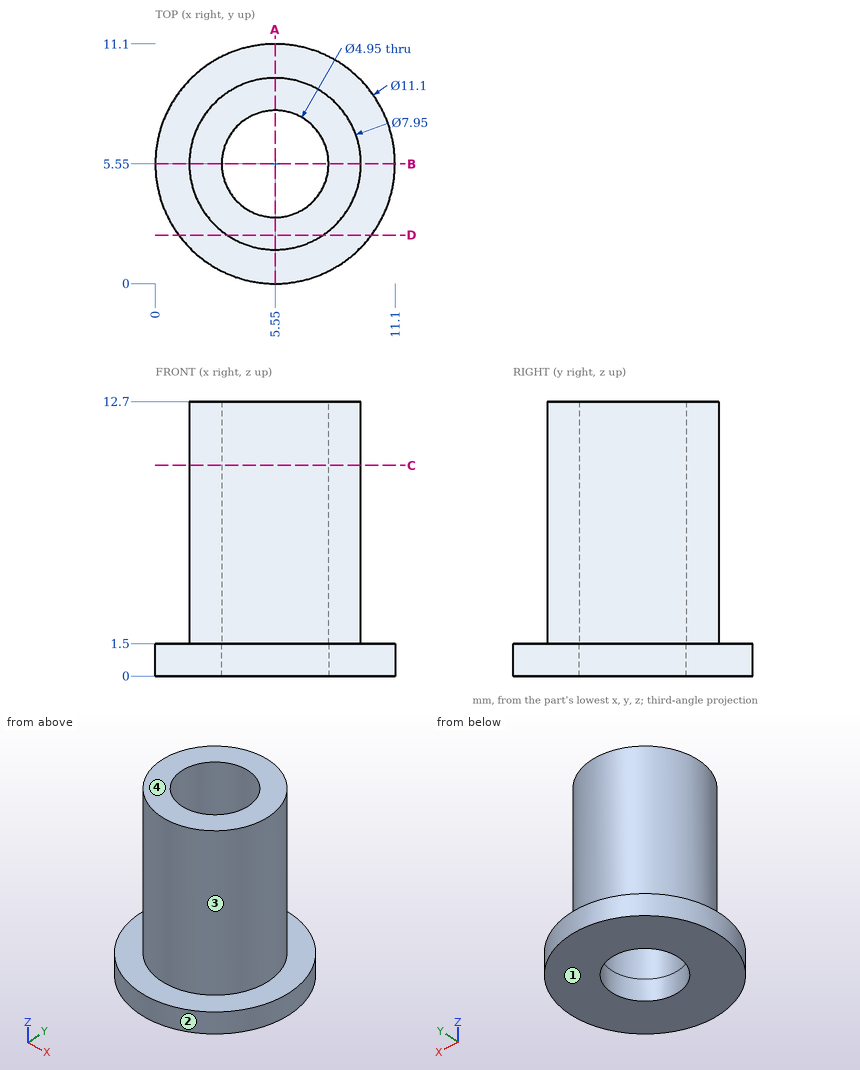
Here's the drawing with two shaded views (mm, measured from the low corner). I have some questions. A direction names the side the tool comes from. Coordinates: 2 decimals unless noted, no trailing zeros. Loops run counter-clockwise (first coordinate to the right, second up) from the corner with the lowest first, then second, coordinate; pieces in that order, holes last. Notation, with made-up numbers: (6.25, -4.75) -> (64.25, -4.75) arc R18 ccw to (64.25, 0.25) -> close; hole circle Ø11 at (62.25, 50.25). An arc over 180 degrees is marked (long way). Use one line per item in the form item = value. Start each with the question number.
(1) If we section it at D-D (y = 2.25): Please give me the cut outline in (x, z).
(2) Please list where these lines run through material, in increasing order: line 1 along Y through (x, z) = (5.55, 5.5) (3 decimals); line 2 along Y through (x, z) = (5.55, 0.4) (3 decimals); line 3 along Z through (x, y) = (2, 8).
(3) We'd pull the mould along X, two halves only. Please class the marked faces 1 and 2: pulls with the +X half, pulls with the -X half, needs draft (parallel to the pull), parting line crosses it, or undercut.
(4) If we section it at A-A (x = 5.55): Please give me the cut outline in (y, z) (3 decimals).
(5) On a 3-axis mill with a long thin cutter (end or side, diameter ignored), from which of +Z, -Z, +X, -X, +Y, -Y can I reach the whole of each face in a straight line? I mean the marked faces 3 and 4. Say none if no direction works.
(6) Will these pins go through, and if not, where does the flat tip stop? pin 1 (6 mm diameter, centred on x = 9, y = 6, fed in from -Z); pin 2 (1 mm diameter, centred on x = 2.5, z = 2.5, fed in from +Y); pin 3 (6 mm diameter, centred on y = 6.5, z = 7.5, fed in from +X) (3 decimals); pin 4 (1 mm diameter, centred on y = 9, z = 7.5, fed in from +X).
(7) If we section it at C-C (z = 9.75): Please give me the cut outline in (x, y) (3 decimals).
Verdict:
q1.outline = (1.09, 0) -> (10.01, 0) -> (10.01, 1.5) -> (7.77, 1.5) -> (7.77, 12.7) -> (3.33, 12.7) -> (3.33, 1.5) -> (1.09, 1.5) -> close
q2.line_1 = 1.575 to 3.075, 8.025 to 9.525
q2.line_2 = 0 to 3.075, 8.025 to 11.1
q2.line_3 = 0 to 1.5
q3.face_1 = needs draft
q3.face_2 = parting line crosses it
q4.outline = (0, 0) -> (3.075, 0) -> (3.075, 12.7) -> (1.575, 12.7) -> (1.575, 1.5) -> (0, 1.5) -> close; (8.025, 0) -> (11.1, 0) -> (11.1, 1.5) -> (9.525, 1.5) -> (9.525, 12.7) -> (8.025, 12.7) -> close
q5.face_3 = +Z
q5.face_4 = +Z, +X, -X, +Y, -Y
q6.pin_1 = 0
q6.pin_2 = 8.6
q6.pin_3 = 9.525
q6.pin_4 = 8.21
q7.outline = circle Ø7.95 at (5.55, 5.55); hole circle Ø4.95 at (5.55, 5.55)
